For this review, take the finished solid that the model builds, in its own axes (mm). A direction names the side the tool comes from. Give positions to 0.01 mm unless a question says otherwise; leave off trailing zeros. Order: outer loops, then holes, each group sorted by start corner. A loop starts at its lowest first (then second) coordinate and runs counter-clockwise, first axis right, second up. Notation, with made-up numbers: (5, -25) -> (21, -25) arc R27 cw to (21, 10) -> close; hole circle Ø2 at (64, 8.25). An arc over 180 degrees is marked (long way). Use CSV: the item, a comma, the result in double quotes. Start each with the question number.
```python
from build123d import *
from OCP.BRepFilletAPI import BRepFilletAPI_MakeChamfer

# Parameters (mm, degrees)
SKETCH1_W                      = 120
SKETCH1_H                      = 120
BOSS_EXTRUDE1_DEPTH            = 80
CHAMFER1_SIZE                  = 15
SKETCH2_R                      = 8
SKETCH2_R_2                    = 16
CUT_EXTRUDE1_DEPTH             = 80
CUT_EXTRUDE2_DEPTH             = 8
CHAMFER3_SIZE                  = 13.856406461
CHAMFER3_SIZE_2                = 8
CIRPATTERN2_COUNT              = 4
CHAMFER3_OF_CIRPATTERN2_SIZE   = 13.856406461
CHAMFER3_OF_CIRPATTERN2_SIZE_2 = 8
BOSS_EXTRUDE2_START            = 12
SKETCH5_R                      = 40
SKETCH5_R_2                    = 16
BOSS_EXTRUDE2_DEPTH            = 12
SKETCH6_R                      = 32.5
CUT_EXTRUDE3_DEPTH             = 25
BOSS_EXTRUDE3_START            = 4
SKETCH17_R                     = 38.5
SKETCH17_R_2                   = 32.5
BOSS_EXTRUDE3_DEPTH            = 4
CUT_EXTRUDE4_DEPTH             = 156


with BuildPart() as part:
    # Sketch1 → Boss-Extrude1 (new body)
    with BuildSketch(Plane(origin=(0, 0, 0), x_dir=(1, 0, 0), z_dir=(0, 1, 0))):
        Rectangle(SKETCH1_W, SKETCH1_H)
    extrude(amount=BOSS_EXTRUDE1_DEPTH)

    # Chamfer1
    chamfer1_edges = [part.edges().sort_by_distance(p)[0] for p in [
        (60, 40, 60),
        (-60, 40, 60),
        (-60, 40, -60),
        (60, 40, -60),
    ]]
    chamfer(chamfer1_edges, length=CHAMFER1_SIZE)

    # Sketch2 → Cut-Extrude1 (cut)
    with BuildSketch(Plane(origin=(0, 80, 0), x_dir=(1, 0, 0), z_dir=(0, 1, 0))):
        with Locations(Location((-40.658639918, 40.658639918, 0), (0, 0, 270))):
            Circle(SKETCH2_R)
        with Locations(Location((40.658639918, 40.658639918, 0), (0, 0, 270))):
            Circle(SKETCH2_R)
        with Locations(Location((40.658639918, -40.658639918, 0), (0, 0, 270))):
            Circle(SKETCH2_R)
        with Locations(Location((-40.658639918, -40.658639918, 0), (0, 0, 270))):
            Circle(SKETCH2_R)
        with Locations(Location((0, 0, 0), (0, 0, 270))):
            Circle(SKETCH2_R_2)
    extrude(amount=-CUT_EXTRUDE1_DEPTH, mode=Mode.SUBTRACT)

    # Sketch3 → Cut-Extrude2 (cut)
    with BuildSketch(Plane(origin=(60, 0, 0), x_dir=(0, 0, -1), z_dir=(1, 0, 0))):
        with BuildLine():
            Line((-21.061459243, 25), (-21.061459243, 0))
            Line((-21.061459243, 0), (0, 0))
            Line((0, 0), (0, 46.061459243))
            ThreePointArc((0, 46.061459243), (-14.892700652, 39.892700652), (-21.061459243, 25))
        make_face()
        with BuildLine():
            Line((0, 46.061459243), (0, 0))
            Line((0, 0), (21.061459243, 0))
            Line((21.061459243, 0), (21.061459243, 25))
            ThreePointArc((21.061459243, 25), (14.892700652, 39.892700652), (0, 46.061459243))
        make_face()
    cut_extrude2 = extrude(amount=-CUT_EXTRUDE2_DEPTH, mode=Mode.SUBTRACT)

    # Chamfer3
    chamfer3_edges_1 = [part.edges().sort_by_distance(p)[0] for p in [
        (60, 12.5, 21.061459243),
    ]]
    chamfer3_side_1 = [part.faces().sort_by_distance(p)[0] for p in [
        (60, 12.5, 21.221459243),
    ]]
    chamfer3_edges_2 = [part.edges().sort_by_distance(p)[0] for p in [
        (60, 46.061459243, 0),
    ]]
    chamfer3_side_2 = [part.faces().sort_by_distance(p)[0] for p in [
        (60, 46.221459243, 0),
    ]]
    chamfer3_edges_3 = [part.edges().sort_by_distance(p)[0] for p in [
        (60, 12.5, -21.061459243),
    ]]
    chamfer3_side_3 = [part.faces().sort_by_distance(p)[0] for p in [
        (60, 12.5, -21.221459243),
    ]]
    chamfer3 = BRepFilletAPI_MakeChamfer(part.part.solid().wrapped)
    for e in chamfer3_edges_1:
        chamfer3.Add(CHAMFER3_SIZE - 0.0001, CHAMFER3_SIZE_2 - 0.0001, e.wrapped, chamfer3_side_1[0].wrapped)
    for e in chamfer3_edges_2:
        chamfer3.Add(CHAMFER3_SIZE - 0.0001, CHAMFER3_SIZE_2 - 0.0001, e.wrapped, chamfer3_side_2[0].wrapped)
    for e in chamfer3_edges_3:
        chamfer3.Add(CHAMFER3_SIZE - 0.0001, CHAMFER3_SIZE_2 - 0.0001, e.wrapped, chamfer3_side_3[0].wrapped)
    add(Compound.cast(chamfer3.Shape()), mode=Mode.REPLACE)  # a hair under: the kernel refuses the full size

    # CirPattern2: Cut-Extrude2 ×4 about axis
    cirpattern2_axis = Axis((0, 0, 0), (0, 1, 0))
    for i in range(1, CIRPATTERN2_COUNT):
        add(cut_extrude2.rotate(cirpattern2_axis, i * 360 / CIRPATTERN2_COUNT), mode=Mode.SUBTRACT)

    # Chamfer3 of CirPattern2
    chamfer3_of_cirpattern2_edges_1 = [part.edges().sort_by_distance(p)[0] for p in [
        (21.061459243, 12.5, -60),
    ]]
    chamfer3_of_cirpattern2_side_1 = [part.faces().sort_by_distance(p)[0] for p in [
        (21.221459243, 12.5, -60),
    ]]
    chamfer3_of_cirpattern2_edges_2 = [part.edges().sort_by_distance(p)[0] for p in [
        (0, 46.061459243, -60),
    ]]
    chamfer3_of_cirpattern2_side_2 = [part.faces().sort_by_distance(p)[0] for p in [
        (0, 46.221459243, -60),
    ]]
    chamfer3_of_cirpattern2_edges_3 = [part.edges().sort_by_distance(p)[0] for p in [
        (-21.061459243, 12.5, -60),
    ]]
    chamfer3_of_cirpattern2_side_3 = [part.faces().sort_by_distance(p)[0] for p in [
        (-21.221459243, 12.5, -60),
    ]]
    chamfer3_of_cirpattern2_edges_4 = [part.edges().sort_by_distance(p)[0] for p in [
        (-60, 12.5, -21.061459243),
    ]]
    chamfer3_of_cirpattern2_side_4 = [part.faces().sort_by_distance(p)[0] for p in [
        (-60, 12.5, -21.221459243),
    ]]
    chamfer3_of_cirpattern2_edges_5 = [part.edges().sort_by_distance(p)[0] for p in [
        (-60, 46.061459243, 0),
    ]]
    chamfer3_of_cirpattern2_side_5 = [part.faces().sort_by_distance(p)[0] for p in [
        (-60, 46.221459243, 0),
    ]]
    chamfer3_of_cirpattern2_edges_6 = [part.edges().sort_by_distance(p)[0] for p in [
        (-60, 12.5, 21.061459243),
    ]]
    chamfer3_of_cirpattern2_side_6 = [part.faces().sort_by_distance(p)[0] for p in [
        (-60, 12.5, 21.221459243),
    ]]
    chamfer3_of_cirpattern2_edges_7 = [part.edges().sort_by_distance(p)[0] for p in [
        (-21.061459243, 12.5, 60),
    ]]
    chamfer3_of_cirpattern2_side_7 = [part.faces().sort_by_distance(p)[0] for p in [
        (-21.221459243, 12.5, 60),
    ]]
    chamfer3_of_cirpattern2_edges_8 = [part.edges().sort_by_distance(p)[0] for p in [
        (0, 46.061459243, 60),
    ]]
    chamfer3_of_cirpattern2_side_8 = [part.faces().sort_by_distance(p)[0] for p in [
        (0, 46.221459243, 60),
    ]]
    chamfer3_of_cirpattern2_edges_9 = [part.edges().sort_by_distance(p)[0] for p in [
        (21.061459243, 12.5, 60),
    ]]
    chamfer3_of_cirpattern2_side_9 = [part.faces().sort_by_distance(p)[0] for p in [
        (21.221459243, 12.5, 60),
    ]]
    chamfer3_of_cirpattern2 = BRepFilletAPI_MakeChamfer(part.part.solid().wrapped)
    for e in chamfer3_of_cirpattern2_edges_1:
        chamfer3_of_cirpattern2.Add(CHAMFER3_OF_CIRPATTERN2_SIZE - 0.0001, CHAMFER3_OF_CIRPATTERN2_SIZE_2 - 0.0001, e.wrapped, chamfer3_of_cirpattern2_side_1[0].wrapped)
    for e in chamfer3_of_cirpattern2_edges_2:
        chamfer3_of_cirpattern2.Add(CHAMFER3_OF_CIRPATTERN2_SIZE - 0.0001, CHAMFER3_OF_CIRPATTERN2_SIZE_2 - 0.0001, e.wrapped, chamfer3_of_cirpattern2_side_2[0].wrapped)
    for e in chamfer3_of_cirpattern2_edges_3:
        chamfer3_of_cirpattern2.Add(CHAMFER3_OF_CIRPATTERN2_SIZE - 0.0001, CHAMFER3_OF_CIRPATTERN2_SIZE_2 - 0.0001, e.wrapped, chamfer3_of_cirpattern2_side_3[0].wrapped)
    for e in chamfer3_of_cirpattern2_edges_4:
        chamfer3_of_cirpattern2.Add(CHAMFER3_OF_CIRPATTERN2_SIZE - 0.0001, CHAMFER3_OF_CIRPATTERN2_SIZE_2 - 0.0001, e.wrapped, chamfer3_of_cirpattern2_side_4[0].wrapped)
    for e in chamfer3_of_cirpattern2_edges_5:
        chamfer3_of_cirpattern2.Add(CHAMFER3_OF_CIRPATTERN2_SIZE - 0.0001, CHAMFER3_OF_CIRPATTERN2_SIZE_2 - 0.0001, e.wrapped, chamfer3_of_cirpattern2_side_5[0].wrapped)
    for e in chamfer3_of_cirpattern2_edges_6:
        chamfer3_of_cirpattern2.Add(CHAMFER3_OF_CIRPATTERN2_SIZE - 0.0001, CHAMFER3_OF_CIRPATTERN2_SIZE_2 - 0.0001, e.wrapped, chamfer3_of_cirpattern2_side_6[0].wrapped)
    for e in chamfer3_of_cirpattern2_edges_7:
        chamfer3_of_cirpattern2.Add(CHAMFER3_OF_CIRPATTERN2_SIZE - 0.0001, CHAMFER3_OF_CIRPATTERN2_SIZE_2 - 0.0001, e.wrapped, chamfer3_of_cirpattern2_side_7[0].wrapped)
    for e in chamfer3_of_cirpattern2_edges_8:
        chamfer3_of_cirpattern2.Add(CHAMFER3_OF_CIRPATTERN2_SIZE - 0.0001, CHAMFER3_OF_CIRPATTERN2_SIZE_2 - 0.0001, e.wrapped, chamfer3_of_cirpattern2_side_8[0].wrapped)
    for e in chamfer3_of_cirpattern2_edges_9:
        chamfer3_of_cirpattern2.Add(CHAMFER3_OF_CIRPATTERN2_SIZE - 0.0001, CHAMFER3_OF_CIRPATTERN2_SIZE_2 - 0.0001, e.wrapped, chamfer3_of_cirpattern2_side_9[0].wrapped)
    add(Compound.cast(chamfer3_of_cirpattern2.Shape()), mode=Mode.REPLACE)  # a hair under: the kernel refuses the full size

    # Sketch5 → Boss-Extrude2 (add)
    with BuildSketch(Plane(origin=(0, 80, 0), x_dir=(1, 0, 0), z_dir=(0, 1, 0)).offset(BOSS_EXTRUDE2_START)):
        with Locations(Location((0, 0, 0), (0, 0, 90))):
            Circle(SKETCH5_R)
        with Locations(Location((0, 0, 0), (0, 0, 270))):
            Circle(SKETCH5_R_2, mode=Mode.SUBTRACT)
    extrude(amount=-BOSS_EXTRUDE2_DEPTH)

    # Sketch6 → Cut-Extrude3 (cut)
    with BuildSketch(Plane.XZ):
        with Locations(Location((0, 0, 0), (0, 0, 270))):
            Circle(SKETCH6_R)
    extrude(amount=-CUT_EXTRUDE3_DEPTH, mode=Mode.SUBTRACT)

    # Sketch17 → Boss-Extrude3 (add)
    with BuildSketch(Plane.XZ.offset(BOSS_EXTRUDE3_START)):
        with Locations(Location((0, 0, 0), (0, 0, 270))):
            Circle(SKETCH17_R)
        with Locations(Location((0, 0, 0), (0, 0, 270))):
            Circle(SKETCH17_R_2, mode=Mode.SUBTRACT)
    extrude(amount=-BOSS_EXTRUDE3_DEPTH)

    # Sketch18 → Cut-Extrude4 (cut)
    with BuildSketch(Plane.XY.offset(52)):
        Polygon((9, 4), (0, 4), (0, 0), (11.309401077, 0), align=None)
        Polygon((0, 4), (-9, 4), (-11.309401077, 0), (0, 0), align=None)
        Polygon((0, 0), (-11.309401077, 0), (-13.618802154, -4), (0, -4), align=None)
        Polygon((11.309401077, 0), (0, 0), (0, -4), (13.618802154, -4), align=None)
    extrude(amount=-CUT_EXTRUDE4_DEPTH, mode=Mode.SUBTRACT)


solid = part.part
```
1. To check wall thickness, follow L1, parallel to Z at x = -41, y = 24; L2, parallel to Z at x = 0, y = 18.25; L3, parallel to X at y = 41, z = 0. State the ranges of each line that lie inside material, in increasing order. Write a range as [from, to].
2. Consider section A-A (y = 83). State the section outline as (x, z) points.
3. Draft analysis for pull direction Z (two halves, no side actions). For faces 1 (the face through (-38.494, -2.028, 0.686)), 2 (the face through (-52, 23, 0)), 3 (the face through (52, 23, 0)), 4 (the face through (-10.764, 0.945, -40.597)), state which applies: +Z half, -Z half, draft (parallel to the pull), parting line (faces both ways), or undercut.
4. Clearance check with flat-ended pins moving along their axes: P1, Ø8, axis at x = -11.5, z = -41, coming from the -Y side; P2, Ø4, axis at x = 46, z = -45.5, coming from the +Y side; P3, Ø6, axis at y = 21.5, z = -31, coming from the -X side. State where each tip first meets the part, or that it passes through.
5. For faces 5 (the face through (0, 4, -41)), 6 (the face through (0, 23, 52)), 7 (the face through (38.494, -2.028, -0.686)), list the 3-axis set-ups (+Z, -Z, +X, -X, +Y, -Y) from which the entire face can be reached by the end or side of a thin tool; tool diameter is ignored.
6. Consider section B-B (y = 16). State how many separate pieces and enclosed holes the cut face has, plus the area to 3 significant figures.
Answer list:
1,L1,"[-60, -48.65], [-32.67, 32.67], [48.65, 60]"
1,L2,"[-52, -32.5], [32.5, 52]"
1,L3,"[-52, -16], [16, 52]"
2,outline,"circle Ø80 at (0, 0); hole circle Ø32 at (0, 0)"
3,face 1,"parting line"
3,face 2,"undercut"
3,face 3,"undercut"
3,face 4,"draft"
4,P1,"y = 0"
4,P2,"y = 80"
4,P3,"x = -59.47"
5,face 5,"+Z, -Z, -Y"
5,face 6,"+Z, -Y"
5,face 7,"+X, -Y"
6,separate pieces,"1"
6,enclosed holes,"5"
6,area,"8,040 mm2"
